Source: three-view drawing plus pictorial views. Frame: mm from the lowest corner of the part. Give positions to 0.01 mm unless a question says otherwise; leave off trailing zeros. Loops run counter-clockwise (first coordinate to the right, second up) from the corner with the lowest first, then second, coordinate; pieces in that order, holes last.
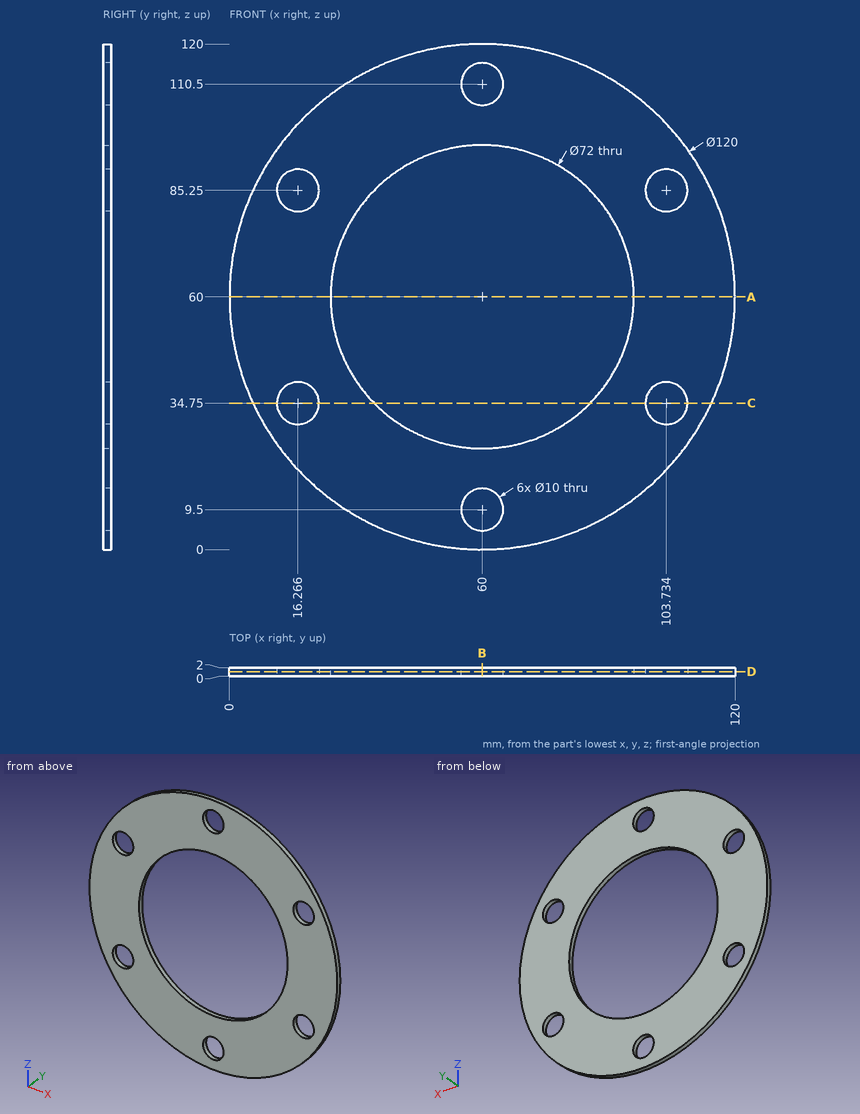
1) Cut plane D-D (y = 1.05). Return loops of the section in (x, z), and give its area (3 significant figures).
Checks:
outline: circle Ø120 at (60, 60); hole circle Ø10 at (16.27, 34.75); hole circle Ø10 at (16.27, 85.25); hole circle Ø72 at (60, 60); hole circle Ø10 at (60, 9.5); hole circle Ø10 at (60, 110.5); hole circle Ø10 at (103.73, 34.75); hole circle Ø10 at (103.73, 85.25)
area: 6,770 mm2
2) Cut plane B-B (x = 60). Return loops of the section in (y, z), and give its area (3 significant figures).
Checks:
outline: (0, 0) - (2, 0) - (2, 4.5) - (0, 4.5) - close; (0, 14.5) - (2, 14.5) - (2, 24) - (0, 24) - close; (0, 96) - (2, 96) - (2, 105.5) - (0, 105.5) - close; (0, 115.5) - (2, 115.5) - (2, 120) - (0, 120) - close
area: 56.0 mm2
3) Cut plane C-C (z = 34.75). Return loops of the section in (x, y).
Checks:
outline: (5.57, 0) - (11.27, 0) - (11.27, 2) - (5.57, 2) - close; (21.27, 0) - (34.34, 0) - (34.34, 2) - (21.27, 2) - close; (85.66, 0) - (98.73, 0) - (98.73, 2) - (85.66, 2) - close; (108.73, 0) - (114.43, 0) - (114.43, 2) - (108.73, 2) - close
4) Contact query for a flat-ended pin moving along its axis: P1, Ø1, axis at x = 40.5, y = 0.5, coming from the -Z side. Output: stop coordinate, or through.
Checks:
P1: stops at z = 3.09
5) Ray query, probe 1 along Z at (x, y) = (60, 1.2); probe 2 along X at (y, z) = (0.8, 86) (1 decimal); probe 3 along X at (y, z) = (1.6, 34.75) (1 decimal). Return the intervals inside material, ascending.
Checks:
probe 1: z = 0 to 4.5, 14.5 to 24, 96 to 105.5, 115.5 to 120
probe 2: x = 5.9 to 11.3, 21.2 to 35.1, 84.9 to 98.8, 108.7 to 114.1
probe 3: x = 5.6 to 11.3, 21.3 to 34.3, 85.7 to 98.7, 108.7 to 114.4
6) Cut plane A-A (z = 60). Return loops of the section in (x, y).
Checks:
outline: (0, 0) - (24, 0) - (24, 2) - (0, 2) - close; (96, 0) - (120, 0) - (120, 2) - (96, 2) - close
